Build history of the part. All positions in model axes, mm. Give positions to 0.01 mm unless a question says otherwise; leave off trailing zeros. Loops run counter-clockwise (first coordinate to the right, second up) from the corner with the lowest first, then second, coordinate; pieces in that order, holes last. Notation, with made-up numbers: M -11,-1.75 L 1,-1.75 A28 cw 1,20.25 Z; hole C 35,39.25 d3. An arc over 180 degrees is marked long. Answer in a Markdown table with one row per item. Add a question column.
```python
from build123d import *

# Parameters (mm, degrees)
CHAMFER_1_SIZE = 0.5


with BuildPart() as part:
    # Эскиз1 → Повернуть1 (revolve)
    with BuildSketch(Plane.XY, mode=Mode.PRIVATE) as revolve_1_sk:
        Polygon((0, 9), (0, 12), (60, 12), (60, 15), (63, 15), (63, 9), align=None)
    revolve(revolve_1_sk.sketch.rotate(Axis((0, 0, 0), (1, 0, 0)), 180), axis=Axis((0, 0, 0), (1, 0, 0)))

    # Фаска1
    chamfer_1_edges = [part.edges().sort_by_distance(p)[0] for p in [
        (60, 15, 0),
        (0, 12, 0),
        (0, 9, 0),
        (63, 9, 0),
        (63, 15, 0),
    ]]
    chamfer(chamfer_1_edges, length=CHAMFER_1_SIZE)


solid = part.part
```
(1) Pin check, flat tips, straight feed: pin 1 (12 mm diameter, centred on x = 30.5, y = -4.5, fed in from -Z); pin 2 (12 mm diameter, centred on x = 54.5, y = 5.5, fed in from -Z); pin 3 (11 mm diameter, centred on y = 0, z = 0, fed in from -X); pin 4 (8 mm diameter, centred on x = 17.5, y = -3.5, fed in from +Z). Stop position of each tip, or through.
(2) Pull direction Y, two halves, no side cores. Call faces 1 (the flat face through (60, 2, -12)), 2 (the cylindrical face through (31.066, 6.633, -6.083)), 3 (the cylindrical face through (30.666, -11.446, -3.604)): +Y half, -Y half, draft (parallel to the pull), parting line (faces both ways), or undercut.
(3) Slice it at A-A, the plane y = 0. Give the cut face in (x, z), then the cut area to 3 significant figures.
(4) Slice it at C-C, the plane x = 52. Give the cut face in (y, z).
(5) Wall check: line 1 (Z direction, x = 52.5, y = -0.5); line 2 (X direction, y = 8, z = -9). Give the ranges that are in metal, low to high.
Solution:
| question | item | result |
|---|---|---|
| 1 | pin 1 | z = -12 |
| 1 | pin 2 | z = -14.26 |
| 1 | pin 3 | through |
| 1 | pin 4 | z = 12 |
| 2 | face 1 | draft |
| 2 | face 2 | undercut |
| 2 | face 3 | parting line |
| 3 | outline | M 0,-11.5 L 0.5,-12 L 60,-12 L 60,-14.5 L 60.5,-15 L 62.5,-15 L 63,-14.5 L 63,-9.5 L 62.5,-9 L 0.5,-9 L 0,-9.5 Z; M 0,9.5 L 0.5,9 L 62.5,9 L 63,9.5 L 63,14.5 L 62.5,15 L 60.5,15 L 60,14.5 L 60,12 L 0.5,12 L 0,11.5 Z |
| 3 | area | 395 mm^2 |
| 4 | outline | C 0,0 d24; hole C 0,0 d18 |
| 5 | line 1 | -11.99 to -8.99, 8.99 to 11.99 |
| 5 | line 2 | 60 to 63 |
